from build123d import *

# Parameters (mm, degrees)
SKETCH1_W           = 62
SKETCH1_H           = 62
SKETCH1_R           = 1.5
BOSS_EXTRUDE1_DEPTH = 10
SKETCH2_R           = 1.5
CUT_EXTRUDE1_DEPTH  = 10
SKETCH3_R           = 1.5
CUT_EXTRUDE2_DEPTH  = 10
SKETCH4_R           = 5
SKETCH4_R_2         = 1.5
CUT_EXTRUDE3_DEPTH  = 10


with BuildPart() as part:
    # Sketch1 → Boss-Extrude1 (new body)
    with BuildSketch(Plane.XY):
        Rectangle(SKETCH1_W, SKETCH1_H)
        with Locations((0, 16.5)):
            Circle(SKETCH1_R, mode=Mode.SUBTRACT)
        with Locations((16.5, 0)):
            Circle(SKETCH1_R, mode=Mode.SUBTRACT)
        with Locations((0, -16.5)):
            Circle(SKETCH1_R, mode=Mode.SUBTRACT)
        with Locations((-16.5, 0)):
            Circle(SKETCH1_R, mode=Mode.SUBTRACT)
    extrude(amount=BOSS_EXTRUDE1_DEPTH)

    # Sketch2 → Cut-Extrude1 (cut)
    with BuildSketch(Plane(origin=(0, 0, 0), x_dir=(-1, 0, 0), z_dir=(0, 0, -1))):
        with Locations((-12.197591975, 12.197591975)):
            Circle(SKETCH2_R)
        with Locations((-12.197591975, -12.197591975)):
            Circle(SKETCH2_R)
        with Locations((12.197591975, -12.197591975)):
            Circle(SKETCH2_R)
        with Locations((12.197591975, 12.197591975)):
            Circle(SKETCH2_R)
    extrude(amount=-CUT_EXTRUDE1_DEPTH, mode=Mode.SUBTRACT)

    # Sketch3 → Cut-Extrude2 (cut)
    with BuildSketch(Plane(origin=(0, 0, 0), x_dir=(-1, 0, 0), z_dir=(0, 0, -1))):
        with Locations((-26, 0)):
            Circle(SKETCH3_R)
        with Locations((0, 26)):
            Circle(SKETCH3_R)
        with Locations((26, 0)):
            Circle(SKETCH3_R)
        with Locations((0, -26)):
            Circle(SKETCH3_R)
    extrude(amount=-CUT_EXTRUDE2_DEPTH, mode=Mode.SUBTRACT)

    # Sketch4 → Cut-Extrude3 (cut)
    with BuildSketch(Plane(origin=(0, 0, 0), x_dir=(-1, 0, 0), z_dir=(0, 0, -1))):
        Circle(SKETCH4_R)
        with Locations((-19.798989873, 19.798989873)):
            Circle(SKETCH4_R_2)
        with Locations((19.798989873, 19.798989873)):
            Circle(SKETCH4_R_2)
        with Locations((19.798989873, -19.798989873)):
            Circle(SKETCH4_R_2)
        with Locations((-19.798989873, -19.798989873)):
            Circle(SKETCH4_R_2)
    extrude(amount=-CUT_EXTRUDE3_DEPTH, mode=Mode.SUBTRACT)


solid = part.part
Check sheet for the modelled part. Datum: model origin and axes. Units: mm. Round coordinates to 2 decimals unless told otherwise and drop trailing zeros. Loops run counter-clockwise (first coordinate to the right, second up) from the corner with the lowest first, then second, coordinate; pieces in that order, holes last.
1. Sectioned sample at B-B on y = 0. Record the boundary of the cut face in (x, z), and give its area (3 significant figures).
2. Gauge pin test, flat ends, axial feed: pin 1 Ø10 at (x, y) = (3, 15) entering from -Z; pin 2 Ø8 at (x, y) = (0, 0) entering from -Z. Record the tip position at first contact, or that the pin passes through.
3. Sectioned sample at D-D on x = -20.5. Record the boundary of the cut face in (y, z).
4. Sectioned sample at A-A on x = 26. Record the boundary of the cut face in (y, z), and give its area (3 significant figures).
5. Mould release check, pull along X, two halves, no side actions. Record for faces 1 (the cylindrical face through (0, -18, 5)), 2 (the flat face through (31, 0, 5)), 3 (the flat face through (0, -31, 5)): released by +X, released by -X, zero draft, split by the parting line, or undercut.
6. Scan lines: probe 1 along Y at (x, z) = (0, 6); probe 2 along Y at (x, z) = (20, 9); probe 3 along Y at (x, z) = (-21, 6.25). Record each from-to range of solid material in increasing order.
Recorded:
1. outline: (-31, 0) - (-27.5, 0) - (-27.5, 10) - (-31, 10) - close; (-24.5, 0) - (-18, 0) - (-18, 10) - (-24.5, 10) - close; (-15, 0) - (-5, 0) - (-5, 10) - (-15, 10) - close; (5, 0) - (15, 0) - (15, 10) - (5, 10) - close; (18, 0) - (24.5, 0) - (24.5, 10) - (18, 10) - close; (27.5, 0) - (31, 0) - (31, 10) - (27.5, 10) - close
1. area: 400 mm2
2. pin 1: stops at z = 0
2. pin 2: passes through
3. outline: (-31, 0) - (-21.13, 0) - (-21.13, 10) - (-31, 10) - close; (-18.47, 0) - (18.47, 0) - (18.47, 10) - (-18.47, 10) - close; (21.13, 0) - (31, 0) - (31, 10) - (21.13, 10) - close
4. outline: (-31, 0) - (-1.5, 0) - (-1.5, 10) - (-31, 10) - close; (1.5, 0) - (31, 0) - (31, 10) - (1.5, 10) - close
4. area: 590 mm2
5. face 1: undercut
5. face 2: released by +X
5. face 3: zero draft
6. probe 1: y = -31 to -27.5, -24.5 to -18, -15 to -5, 5 to 15, 18 to 24.5, 27.5 to 31
6. probe 2: y = -31 to -21.29, -18.31 to 18.31, 21.29 to 31
6. probe 3: y = -31 to -20.7, -18.9 to 18.9, 20.7 to 31
